Check sheet for the drawn part. Datum: minimum x, y, z corner. Units: mm. Coordinates: 2 decimals unless noted, no trailing zeros. Write each loop counter-clockwise with the first axis right and the second up, starting at its lowest first coordinate (ties: lowest second). Pieces come first, ordered by that corner, then holes. Notation, with made-up numbers: (28.25, -2.75) -> (65.25, -2.75) arc R34 ccw to (65.25, 36.25) -> close; hole circle Ø9 at (55.5, 66). An arc over 180 degrees is marked (long way). Answer in a Markdown table with one row per item. Add a question column.
1. Depth check by flat-ended pin: P1, Ø1.2, axis at y = 1.5, z = 57, coming from the -X side; P2, Ø2, axis at x = 11, y = 2, coming from the +Z side; P3, Ø1.2, axis at x = 48, y = 2.5, coming from the +Z side; P4, Ø6, axis at x = 20, z = 47.5, coming from the +Y side. Enter the tip coordinate at first touch or a pass-through.
2. Scan lines: L1, parallel to X at y = 2.2, z = 47.5; L2, parallel to X at y = 0.95, z = 41.5; L3, parallel to X at y = 3.65, z = 39. Record each from-to range of solid material in increasing order. Write a range as from..to.
3. Cross-section at B-B on y = 1.25. Record the cut outline in (x, z).
4. Cross-section at A-A on z = 47.5. Record the cut outline in (x, y).
5. Cross-section at D-D on z = 74.5. Record the cut outline in (x, y), and give its area (3 significant figures).
6. Cross-section at C-C on x = 20. Record the cut outline in (y, z), and give its area (3 significant figures).
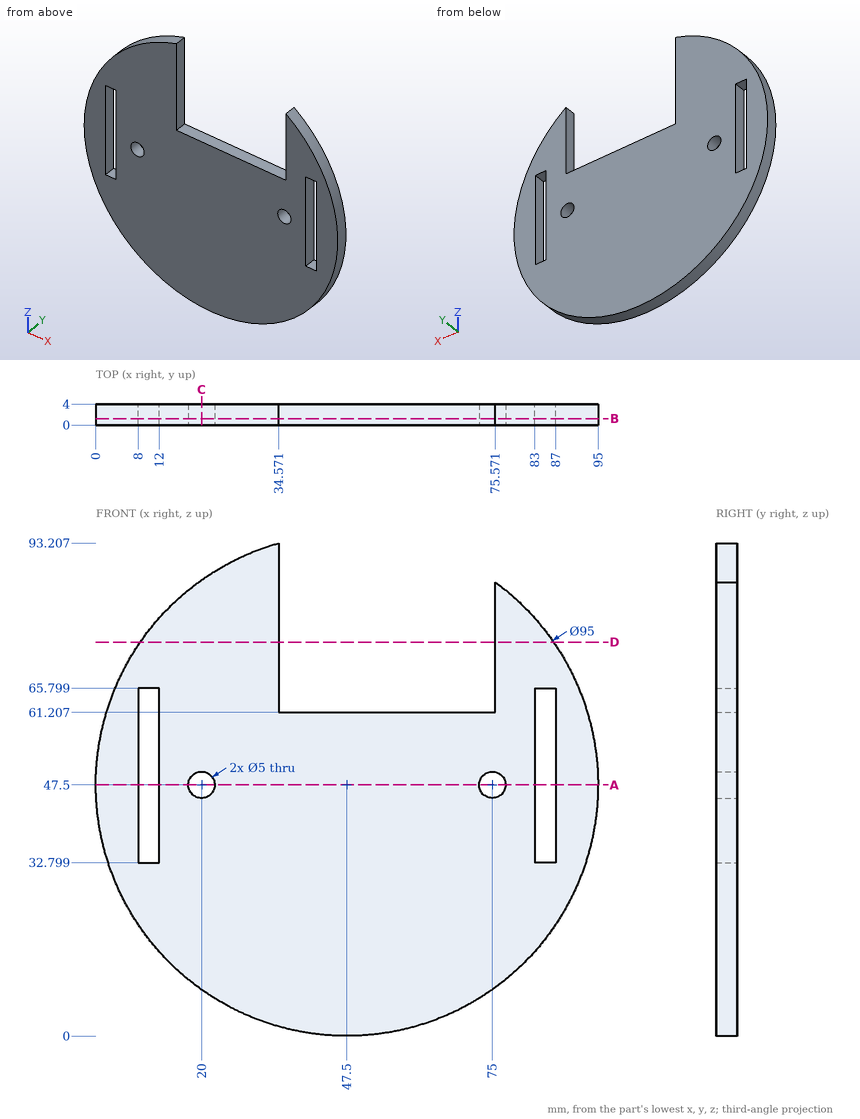
Results found:
| question | item | result |
|---|---|---|
| 1 | P1 | stops at x = 0.84 |
| 1 | P2 | stops at z = 79.06 |
| 1 | P3 | stops at z = 61.21 |
| 1 | P4 | stops at y = 4 |
| 2 | L1 | x = 0..8, 12..17.5, 22.5..72.5, 77.5..83, 87..95 |
| 2 | L2 | x = 0.38..8, 12..83, 87..94.62 |
| 2 | L3 | x = 0.77..8, 12..83, 87..94.23 |
| 3 | outline | (34.57, 61.21) -> (34.57, 93.21) arc R47.5 ccw (long way) to (75.57, 85.82) -> (75.57, 61.21) -> close; hole (8, 32.8) -> (12, 32.8) -> (12, 65.8) -> (8, 65.8) -> close; hole circle Ø5 at (20, 47.5); hole circle Ø5 at (75, 47.5); hole (83, 32.8) -> (87, 32.8) -> (87, 65.8) -> (83, 65.8) -> close |
| 4 | outline | (0, 0) -> (8, 0) -> (8, 4) -> (0, 4) -> close; (12, 0) -> (17.5, 0) -> (17.5, 4) -> (12, 4) -> close; (22.5, 0) -> (72.5, 0) -> (72.5, 4) -> (22.5, 4) -> close; (77.5, 0) -> (83, 0) -> (83, 4) -> (77.5, 4) -> close; (87, 0) -> (95, 0) -> (95, 4) -> (87, 4) -> close |
| 5 | outline | (8.42, 0) -> (34.57, 0) -> (34.57, 4) -> (8.42, 4) -> close; (75.57, 0) -> (86.58, 0) -> (86.58, 4) -> (75.57, 4) -> close |
| 5 | area | 149 mm^2 |
| 6 | outline | (0, 8.77) -> (4, 8.77) -> (4, 45) -> (0, 45) -> close; (0, 50) -> (4, 50) -> (4, 86.23) -> (0, 86.23) -> close |
| 6 | area | 290 mm^2 |
